from build123d import *

# Parameters (mm, degrees)
BOSS_EXTRUDE1_DEPTH       = 160
SHELL4_START              = 2
SHELL4_DEPTH              = 156
SKETCH5_R                 = 90
CUT_EXTRUDE1_DEPTH        = 118
SKETCH6_R                 = 185
BOSS_EXTRUDE2_DEPTH       = 55
BOSS_EXTRUDE2_TAPER       = 51
SKETCH7_R                 = 117.080656391
BOSS_EXTRUDE3_DEPTH       = 10
SKETCH9_R                 = 100
CUT_EXTRUDE2_DEPTH        = 118
SKETCH11_R                = 10
CUT_EXTRUDE3_DEPTH        = 118
SKETCH12_W                = 280
SKETCH12_H                = 240
SKETCH12_W_2              = 196
SKETCH12_H_2              = 156
BOSS_EXTRUDE4_DEPTH       = 10
EXTRUDE_THIN1_OUTLINE_W   = 50
EXTRUDE_THIN1_OUTLINE_H   = 50
EXTRUDE_THIN1_OUTLINE_W_2 = 46
EXTRUDE_THIN1_OUTLINE_H_2 = 46
EXTRUDE_THIN1_DEPTH       = 230
BOSS_EXTRUDE6_START       = 230
SKETCH15_W                = 126
SKETCH15_H                = 128
SKETCH15_W_2              = 128
SKETCH15_H_2              = 126
BOSS_EXTRUDE6_DEPTH       = 10


# Read off the part's stored shape, not the designer's step: Shell4, Extrude-Thin1
with BuildPart() as part:
    # Sketch1 → Boss-Extrude1 (new body)
    with BuildSketch(Plane.XY):
        with BuildLine():
            Line((-181.424802111, -189.973614776), (-181.424802111, 184.026385224))
            Line((-181.424802111, 184.026385224), (18.575197889, 184.026385224))
            Line((18.575197889, 184.026385224), (18.575197889, 140.026385224))
            Line((18.575197889, 140.026385224), (258.575197889, 140.026385224))
            ThreePointArc((258.575197889, 140.026385224), (502.757506831, 45.043449524), (618.575197889, -189.973614776))
            ThreePointArc((618.575197889, -189.973614776), (515.322398935, -459.046095717), (258.575197889, -589.973614776))
            ThreePointArc((258.575197889, -589.973614776), (-38.746177057, -475.027127217), (-181.424802111, -189.973614776))
        make_face()
    extrude(amount=BOSS_EXTRUDE1_DEPTH)

    # Shell4 outline → Shell4 (cut)
    with BuildSketch(Plane.XY.offset(SHELL4_START)):
        with BuildLine():
            ThreePointArc((-179.424802111, -189.878268455), (-37.404584917, -473.543834805), (258.469922203, -587.973602181))
            ThreePointArc((258.469922203, -587.973602181), (513.841925832, -457.701371443), (616.57518844, -190.060584018))
            ThreePointArc((616.57518844, -190.060584018), (501.374009985, 43.598514633), (258.575197889, 138.026385224))
            Line((258.575197889, 138.026385224), (16.575197889, 138.026385224))
            Line((16.575197889, 138.026385224), (16.575197889, 184.026385224))
            Line((16.575197889, 184.026385224), (-179.424802111, 184.026385224))
            Line((-179.424802111, 184.026385224), (-179.424802111, -189.878268455))
        make_face()
    extrude(amount=SHELL4_DEPTH, mode=Mode.SUBTRACT)

    # Sketch5 → Cut-Extrude1 (cut)
    with BuildSketch(Plane.XY.offset(160)):
        with Locations((258.575197889, -189.973614776)):
            Circle(SKETCH5_R)
    extrude(amount=-CUT_EXTRUDE1_DEPTH, mode=Mode.SUBTRACT)

    # Sketch6 → Boss-Extrude2 (add)
    with BuildSketch(Plane.XY.offset(160)):
        with Locations((258.575197889, -189.973614776)):
            Circle(SKETCH6_R)
    extrude(amount=BOSS_EXTRUDE2_DEPTH, taper=BOSS_EXTRUDE2_TAPER)

    # Sketch7 → Boss-Extrude3 (add)
    with BuildSketch(Plane.XY.offset(215)):
        with Locations((258.575197889, -189.973614776)):
            Circle(SKETCH7_R)
    extrude(amount=BOSS_EXTRUDE3_DEPTH)

    # Sketch9 → Cut-Extrude2 (cut)
    with BuildSketch(Plane.XY.offset(225)):
        with Locations((258.575197889, -189.973614776)):
            Circle(SKETCH9_R)
    extrude(amount=-CUT_EXTRUDE2_DEPTH, mode=Mode.SUBTRACT)

    # Sketch11 → Cut-Extrude3 (cut)
    with BuildSketch(Plane(origin=(0, 0, 0), x_dir=(-1, 0, 0), z_dir=(0, 0, -1))):
        with Locations((-258.575197889, -189.973614776)):
            Circle(SKETCH11_R)
    extrude(amount=-CUT_EXTRUDE3_DEPTH, mode=Mode.SUBTRACT)

    # Sketch12 → Boss-Extrude4 (add)
    with BuildSketch(Plane(origin=(0, 184.026385224, 0), x_dir=(1, 0, 0), z_dir=(0, 1, 0))):
        with Locations((-81.424802111, -80)):
            Rectangle(SKETCH12_W, SKETCH12_H)
        with Locations((-81.424802111, -80)):
            Rectangle(SKETCH12_W_2, SKETCH12_H_2, mode=Mode.SUBTRACT)
    extrude(amount=BOSS_EXTRUDE4_DEPTH)

    # Extrude-Thin1 outline → Extrude-Thin1 (add)
    # profile 1 of 4: a face of its own
    with BuildSketch(Plane.XY.offset(160)):
        with Locations((-51.424802111, -189.973614776)):
            Rectangle(EXTRUDE_THIN1_OUTLINE_W, EXTRUDE_THIN1_OUTLINE_H)
        with Locations((-51.424802111, -189.973614776)):
            Rectangle(EXTRUDE_THIN1_OUTLINE_W_2, EXTRUDE_THIN1_OUTLINE_H_2, mode=Mode.SUBTRACT)
    # profile 2 of 4: a face of its own
    with BuildSketch(Plane.XY.offset(160)):
        with Locations((568.575197889, -189.973614776)):
            Rectangle(EXTRUDE_THIN1_OUTLINE_W, EXTRUDE_THIN1_OUTLINE_H)
        with Locations((568.575197889, -189.973614776)):
            Rectangle(EXTRUDE_THIN1_OUTLINE_W_2, EXTRUDE_THIN1_OUTLINE_H_2, mode=Mode.SUBTRACT)
    # profile 3 of 4: a face of its own
    with BuildSketch(Plane.XY.offset(160)):
        with Locations((258.575197889, 120.026385224)):
            Rectangle(EXTRUDE_THIN1_OUTLINE_W, EXTRUDE_THIN1_OUTLINE_H)
        with Locations((258.575197889, 120.026385224)):
            Rectangle(EXTRUDE_THIN1_OUTLINE_W_2, EXTRUDE_THIN1_OUTLINE_H_2, mode=Mode.SUBTRACT)
    # profile 4 of 4: a face of its own
    with BuildSketch(Plane.XY.offset(160)):
        with Locations((258.575197889, -499.973614776)):
            Rectangle(EXTRUDE_THIN1_OUTLINE_W, EXTRUDE_THIN1_OUTLINE_H)
        with Locations((258.575197889, -499.973614776)):
            Rectangle(EXTRUDE_THIN1_OUTLINE_W_2, EXTRUDE_THIN1_OUTLINE_H_2, mode=Mode.SUBTRACT)
    extrude(amount=EXTRUDE_THIN1_DEPTH)

    # Sketch15 → Boss-Extrude6 (add)
    with BuildSketch(Plane.XY.offset(160).offset(BOSS_EXTRUDE6_START)):
        with Locations((258.575197889, -498.973614776)):
            Rectangle(SKETCH15_W, SKETCH15_H)
        with Locations((-50.424802111, -189.973614776)):
            Rectangle(SKETCH15_W_2, SKETCH15_H_2)
        with Locations((258.575197889, 119.026385224)):
            Rectangle(SKETCH15_W, SKETCH15_H)
        with Locations((567.575197889, -189.973614776)):
            Rectangle(SKETCH15_W_2, SKETCH15_H_2)
    extrude(amount=BOSS_EXTRUDE6_DEPTH)


solid = part.part
Read the model definition and answer for the solid it produces. Units are mm, in the model's axes. A direction names the side the tool comes from. Round coordinates to 2 decimals unless told otherwise and drop trailing zeros. Loops run counter-clockwise (first coordinate to the right, second up) from the corner with the lowest first, then second, coordinate; pieces in that order, holes last.
Q1. Section D-D on z = 133.5 is taken. Write down the section's boundary in (x, y), and give its area (3 significant figures).
Q2. Section A-A on z = 337 is taken. Give the number of separate pieces and of enclosed holes in the cut face, and give its area (3 significant figures).
Q3. Consider probe 1 along X at (y, z) = (-176.5, 230.5); probe 2 along Y at (x, z) = (-64, 327); probe 3 along Z at (x, y) = (-145, -74). Determine where each line is inside the solid, lowest interval first.
Q4. Section C-C on y = -393.5 is taken. Write down the section's boundary in (x, z), and give its area (3 significant figures).
Q5. Each of these flat-tipped pins is pushed along its axis until it touches: pin 1 (8 mm diameter, centred on x = 171, y = -195, fed in from -Z); pin 2 (15 mm diameter, centred on y = 121, z = 332, fed in from -X); pin 3 (12 mm diameter, centred on y = -502, z = 210, fed in from +X). Where does it stop, or does it pass through?
Q6. Section B-B on x = 34 is taken. Write down the section's boundary in (y, z).
Q7. Determine the mould class of faces 6 (the face through (283.575, -500, 273)), 7 (the face through (286, -498, 390)), 8 (the face through (258, 145.026, 273)) for opening direction Y: released by +Y, released by -Y, zero draft, split by the parting line, or undercut.
Q8. Which of the six approach directions +Z, -Z, +X, -X, +Y, -Y give full straight-line access (tool end or side, diameter ignored) to faces 1 (the face through (18.575, 162, 79)), 2 (the face through (213, -202, 2)), 3 (the face through (258, -474.974, 273)), 4 (the face through (258, 143.026, 273)), 5 (the face through (16.575, 166, 81))?
Output:
1. outline: (-221.42, 184.03) - (-181.42, 184.03) - (-181.42, -189.97) arc R442 ccw to (258.58, -589.97) arc R402.22 ccw to (618.58, -189.97) arc R361.36 ccw to (258.58, 140.03) - (18.58, 140.03) - (18.58, 184.03) - (58.58, 184.03) - (58.58, 194.03) - (16.58, 194.03) - (16.58, 138.03) - (258.58, 138.03) arc R359.36 cw to (616.58, -190.06) arc R400.22 cw to (258.47, -587.97) arc R440 cw to (-179.42, -189.88) - (-179.42, 194.03) - (-221.42, 194.03) - close
1. area: 5,710 mm2
2. separate pieces: 4
2. enclosed holes: 4
2. area: 1,540 mm2
3. probe 1: x = -76.42 to -74.42, -28.42 to -26.42, 543.58 to 545.58, 591.58 to 593.58
3. probe 2: y = -214.97 to -212.97, -166.97 to -164.97
3. probe 3: z = 0 to 2, 158 to 160
4. outline: (-108.96, 0) - (563.28, 0) - (563.28, 160) - (-108.96, 160) - close; hole (-106.55, 2) - (560.96, 2) - (560.96, 158) - (-106.55, 158) - close
4. area: 3,430 mm2
5. pin 1: stops at z = 0
5. pin 2: stops at x = 233.58
5. pin 3: stops at x = 283.58
6. outline: (-528.67, 0) - (140.03, 0) - (140.03, 160) - (-528.67, 160) - close; (184.03, -40) - (194.03, -40) - (194.03, 200) - (184.03, 200) - close; hole (-526.35, 2) - (138.03, 2) - (138.03, 158) - (-526.35, 158) - close
7. face 6: zero draft
7. face 7: undercut
7. face 8: released by +Y
8. face 1: +Z, -Z, +X
8. face 2: none
8. face 3: +X, -X
8. face 4: -Z
8. face 5: +Y
